from build123d import *

# Parameters (mm, degrees)
SKETCH1_W           = 45.72
SKETCH1_H           = 45.72
BOSS_EXTRUDE1_DEPTH = 2.54
SKETCH2_W           = 6.604
SKETCH2_H           = 6.604
BOSS_EXTRUDE2_DEPTH = 25.4
SKETCH5_R           = 2.125
BOSS_EXTRUDE5_DEPTH = 10.3
SKETCH8_R           = 1.525
BOSS_EXTRUDE8_DEPTH = 14.7
SKETCH9_R           = 1.015
BOSS_EXTRUDE9_DEPTH = 8.3
SKETCH7_W           = 6.35
SKETCH7_H           = 8.89
BOSS_EXTRUDE7_DEPTH = 6.35


with BuildPart() as part:
    # Sketch1 → Boss-Extrude1 (new body)
    with BuildSketch(Plane(origin=(0, 0, 0), x_dir=(1, 0, 0), z_dir=(0, 1, 0))):
        Rectangle(SKETCH1_W, SKETCH1_H)
    extrude(amount=BOSS_EXTRUDE1_DEPTH)

    # Sketch2 → Boss-Extrude2 (add)
    with BuildSketch(Plane(origin=(0, 2.54, 0), x_dir=(1, 0, 0), z_dir=(0, 1, 0))):
        with Locations((16.000000004, 16.000000004)):
            Rectangle(SKETCH2_W, SKETCH2_H)
        with Locations((-16.000000004, 16.000000004)):
            Rectangle(SKETCH2_W, SKETCH2_H)
        with Locations((-16.000000004, -16.000000004)):
            Rectangle(SKETCH2_W, SKETCH2_H)
        with Locations((16.000000004, -16.000000004)):
            Rectangle(SKETCH2_W, SKETCH2_H)
    extrude(amount=BOSS_EXTRUDE2_DEPTH)

    # Sketch5 → Boss-Extrude5 (add)
    with BuildSketch(Plane(origin=(0, 27.94, 0), x_dir=(1, 0, 0), z_dir=(0, 1, 0))):
        with Locations(Location((-16.000000004, 16.000000004, 0), (0, 0, 90))):
            Circle(SKETCH5_R)
        with Locations(Location((16.000000004, 16.000000004, 0), (0, 0, 90))):
            Circle(SKETCH5_R)
        with Locations(Location((-16.000000004, -16.000000004, 0), (0, 0, 90))):
            Circle(SKETCH5_R)
        with Locations(Location((16.000000004, -16.000000004, 0), (0, 0, 90))):
            Circle(SKETCH5_R)
    extrude(amount=BOSS_EXTRUDE5_DEPTH)

    # Sketch8 → Boss-Extrude8 (add)
    with BuildSketch(Plane(origin=(0, 38.24, 0), x_dir=(1, 0, 0), z_dir=(0, 1, 0))):
        with Locations(Location((16, 16, 0), (0, 0, 270))):
            Circle(SKETCH8_R)
        with Locations(Location((-16, 16, 0), (0, 0, 90))):
            Circle(SKETCH8_R)
        with Locations(Location((-16, -16, 0), (0, 0, 270))):
            Circle(SKETCH8_R)
        with Locations(Location((16, -16, 0), (0, 0, 90))):
            Circle(SKETCH8_R)
    extrude(amount=BOSS_EXTRUDE8_DEPTH)

    # Sketch9 → Boss-Extrude9 (add)
    with BuildSketch(Plane(origin=(0, 52.94, 0), x_dir=(1, 0, 0), z_dir=(0, 1, 0))):
        with Locations(Location((16, 16, 0), (0, 0, 90))):
            Circle(SKETCH9_R)
        with Locations(Location((-16, 16, 0), (0, 0, 90))):
            Circle(SKETCH9_R)
        with Locations(Location((-16, -16, 0), (0, 0, 90))):
            Circle(SKETCH9_R)
        with Locations(Location((16, -16, 0), (0, 0, 90))):
            Circle(SKETCH9_R)
    extrude(amount=BOSS_EXTRUDE9_DEPTH)

    # Sketch7 → Boss-Extrude7 (add)
    with BuildSketch(Plane.XZ):
        with Locations((-6, 16.256)):
            Rectangle(SKETCH7_W, SKETCH7_H)
        with Locations((-18, 16.256)):
            Rectangle(SKETCH7_W, SKETCH7_H)
        with Locations((6, 16.256)):
            Rectangle(SKETCH7_W, SKETCH7_H)
        with Locations((18, 16.256)):
            Rectangle(SKETCH7_W, SKETCH7_H)
        with Locations((-6, -16.256)):
            Rectangle(SKETCH7_W, SKETCH7_H)
        with Locations((-18, -16.256)):
            Rectangle(SKETCH7_W, SKETCH7_H)
        with Locations((18, -16.256)):
            Rectangle(SKETCH7_W, SKETCH7_H)
        with Locations((6, -16.256)):
            Rectangle(SKETCH7_W, SKETCH7_H)
    extrude(amount=BOSS_EXTRUDE7_DEPTH)


solid = part.part
Model file for the job. Use its own axes, mm. A direction names the side the tool comes from. Give positions to 0.01 mm unless a question says otherwise; leave off trailing zeros. Order: outer loops, then holes, each group sorted by start corner. A loop starts at its lowest first (then second) coordinate and runs counter-clockwise, first axis right, second up. Notation, with made-up numbers: (34, 33.5) -> (38, 33.5) arc R27 cw to (38, 56.5) -> close; hole circle Ø10 at (60.5, 37.25). An arc over 180 degrees is marked (long way). Use CSV: the item, a comma, the result in double quotes.
1. Drill centre lines: line 1 along X through (y, z) = (22.5, 15); line 2 along X through (y, z) = (36.5, -16) (3 decimals). Where is each one in solid material? Low to high. Write a range as from..to.
Outcome:
line 1,"-19.3..-12.7, 12.7..19.3"
line 2,"-18.125..-13.875, 13.875..18.125"
2. Band-saw the part on A-A, the plane y = -2. Count the separate pieces of the cut face and the enclosed holes in it, then the cut area to 3 significant figures.
Outcome:
separate pieces,"8"
enclosed holes,"0"
area,"452 mm²"
3. Band-saw the part on C-C, the plane y = 49.5. Give the cut face in (x, z) (3 decimals), then the cut area to 3 significant figures.
Outcome:
outline,"circle Ø3.05 at (-16, -16); circle Ø3.05 at (-16, 16); circle Ø3.05 at (16, -16); circle Ø3.05 at (16, 16)"
area,"29.2 mm²"
4. Band-saw the part on B-B, the plane x = -0.5. Give the cut face in (y, z).
Outcome:
outline,"(0, -22.86) -> (2.54, -22.86) -> (2.54, 22.86) -> (0, 22.86) -> close"
5. 3-axis set-ups, long thin cutter, end or side, ignore diameter. For faces 1 (the flat face through (-19.302, 15, 16)), 2 (the cylindrical face through (-16.686, 57.032, -15.252)), 3 (the flat face through (16, 15, -12.698)), 4 (the flat face through (-6, -3, 20.701)): which of +Z, -Z, +X, -X, +Y, -Y reach the whole face in a straight line?
Outcome:
face 1,"+Z, -Z, -X, +Y"
face 2,"+Y"
face 3,"+X, -X, +Y"
face 4,"+Z, +X, -X, -Y"
6. Drop flat-ended pins along their axis: pin 1 (5.5 mm diameter, centred on y = 16, z = -15.5, fed in from +X); pin 2 (8 mm diameter, centred on x = -18, z = 6.5, fed in from -Y); pin 3 (1 mm diameter, centred on x = -13, y = 24, fed in from -Z). Give the stop position or say it passes through.
Outcome:
pin 1,"x = 19.3"
pin 2,"y = 0"
pin 3,"z = -19.3"
7. Mould opens along X. For faces 5 (the flat face through (-14.825, -3, 16)), 6 (the flat face through (9.175, -3, 16)), 7 (the flat face through (-18, -3, 11.811)), 8 (the flat face through (-21.175, -3, 16)) say: +X half, -X half, draft (parallel to the pull), parting line (faces both ways), or undercut.
Outcome:
face 5,"undercut"
face 6,"undercut"
face 7,"draft"
face 8,"-X half"
